Model file for the job. Use its own axes, mm. A direction names the side the tool comes from. Round coordinates to 2 decimals unless told otherwise and drop trailing zeros. Loops run counter-clockwise (first coordinate to the right, second up) from the corner with the lowest first, then second, coordinate; pieces in that order, holes last. Notation, with made-up numbers: M -30.75,16 L 14.25,16 A22 cw 14.25,53 Z; hole C 36,70 d5. An arc over 180 degrees is marked long. Use a Markdown table: item, result. Add a question column.
Q1. Pin check, flat tips, straight feed: pin 1 (6 mm diameter, centred on x = 5, z = 50, fed in from -Y); pin 2 (0.6 mm diameter, centred on x = 1, y = 51.5, fed in from -Z); pin 3 (5 mm diameter, centred on y = 97, z = 70.56, fed in from +X). Stop position of each tip, or through.
Q2. Cut at A-A (x = 6). Give the cut face in (y, z).
Q3. Cut at D-D (z = 78.5). Give the cut face in (x, y), plus the area to 3 significant figures.
Q4. Probe line 1 (Y direction, x = 1, z = 70.5); line 2 (Y direction, x = 1.5, z = 53); line 3 (Z direction, x = 6, y = 101). List the from-to ranges inside material, lowest first. Write a range as from..to.
Q5. Cut at B-B (x = 10.5). Give the cut face in (y, z).
Q6. Mould opens along Y. For faces 1 (the face through (3.2, 64.903, 53.5)), 2 (the face through (1, 109.003, 62)), 3 (the face through (5.19, 70.99, 54.22)) say: +Y half, -Y half, draft (parallel to the pull), parting line (faces both ways), or undercut.
Q7. Cut at C-C (y = 74.5). Give the cut face in (x, z).
Q8. Tool access for faces 4 (the face through (0.99, 98.39, 73.22)), 5 (the face through (3.2, 97.003, 53.5)): list every direction of +Z, -Z, +X, -X, +Y, -Y with a clear straight run to the whole face (end or side of a thin tool).
Autodesk Inventor part; units mm, degrees
ref_plane "Work Plane1" through (2, 70.903, 50.5595) normal (0, 1, 0) x (-1, 0, 0)
ref_plane "YZ Plane" through (0, 0, 0) normal (1, 0, 0) x (0, 1, 0)
ref_plane "XZ Plane" through (0, 0, 0) normal (0, 1, 0) x (-1, 0, 0)
sketch "Sketch1" plane through (0, 0, 0) normal (1, 0, 0) x (0, 1, 0)
  line L0 (109.003, 50.5595) -> (32.803, 50.5595)
  line L1 (32.803, 50.5595) -> (32.803, 88.6595)
  line L2 (32.803, 88.6595) -> (109.003, 88.6595)
  line L3 (109.003, 88.6595) -> (109.003, 50.5595)
  line L4 (76.903, 50.5595) -> (97.003, 50.5595)
  line L5 (97.003, 50.5595) -> (97.003, 57.0595)
  line L6 (97.003, 57.0595) -> (76.903, 57.0595)
  line L7 (76.903, 57.0595) -> (76.903, 50.5595)
  line L8 (44.803, 50.5595) -> (64.903, 50.5595)
  line L9 (64.903, 50.5595) -> (64.903, 57.0595)
  line L10 (64.903, 57.0595) -> (44.803, 57.0595)
  line L11 (44.803, 57.0595) -> (44.803, 50.5595)
  circle A0 centre (97.003, 70.5595) radius 3
  circle A1 centre (83.403, 80.5595) radius 3
  line L12 (70.903, 88.6595) -> (70.903, 50.5595) construction
  circle A2 centre (44.803, 70.5595) radius 3
  circle A3 centre (58.403, 80.5595) radius 3
  point P0 (0, 0)
  dimension "d0" = 76.2
  dimension "d1" = 38.1
  dimension "d2" = 6.5
  dimension "d4" = 12
  dimension "d5" = 12
  dimension "d6" = 12
  dimension "d7" = 6
  dimension "d8" = 6
  dimension "d9" = 20
  dimension "d10" = 30
  dimension "d11" = 12.5
  dimension "d12" = 26.1
extrude "Extrusion1" add sketch "Sketch1" along normal blind 2 contours L0 L5 L6 L7 L9 L10 L11 L1 L2 L3
ref_plane "Work Plane1" through (2, 70.903, 50.5595) normal (0, 1, 0) x (-1, 0, 0)
sketch "Sketch2" plane through (0, 109.003, 88.6595) normal (0, 1, 0) x (1, 0, 0)
  line L0 (0, 38.1) -> (0, 0)
  line L1 (0, 0) -> (2, 0)
  line L2 (2, 38.1) -> (2, 0)
  line L3 (0, 38.1) -> (2, 38.1)
  circle A0 centre (6, 38.1) radius 6
  line L4 (0, 38.1) -> (2, 38.1)
  line L5 (0, 38.1) -> (2, 38.1)
  circle A1 centre (6, 38.1) radius 3.75
  point P0 (0, 88.6595)
  point P1 (1.2193, 34.4744)
  point P2 (0, 38.1)
  dimension "d15" = 0
  dimension "d16" = 12
  dimension "d18" = 7.5
  dimension "d23" = 4
extrude "Extrusion2" add sketch "Sketch2" against normal up to surface (12 mm away) contours A0 L2 L3 | L3 L2 A0
mirror "Mirror1" about plane through (2, 70.903, 50.5595) normal (0, 1, 0) of "Extrusion2"
sketch "Sketch3" plane through (0, 76.903, 57.0595) normal (0, 1, 0) x (1, 0, 0)
  line L0 (0, -31.6) -> (2, -31.6)
  line L1 (0, 6.5) -> (2, 6.5)
  line L2 (0, 6.5) -> (2, 6.5)
  line L3 (0, 6.5) -> (0, -31.6)
  line L4 (2, 2.0279) -> (2, -31.6)
  arc A0 (2, 2.0279) -> (0, 6.5) centre (6, 6.5) ccw
  circle A1 centre (6, 6.5) radius 3.75
  circle A2 centre (6, 6.5) radius 3.75
  line L5 (0, 6.5) -> (0, -31.6)
  line L6 (0, -31.6) -> (2, -31.6)
  line L7 (2, 2.0279) -> (2, -31.6)
  arc A3 (2, 2.0279) -> (0, 6.5) centre (6, 6.5) ccw
  line L8 (2, 6.5) -> (2, 0)
  point P0 (0, 57.0595)
extrude "Extrusion3" add sketch "Sketch3" against normal up to surface (12 mm away) contours A0 L8 L1
equation "\"d5\" = d4"
equation "\"d6\" = d4"
equation "\"d8\" = d7"
properties part number "zawias-lewy" material "Stainless Steel"
Checked values:
| question | item | result |
|---|---|---|
| 1 | pin 1 | stops at y = 32.8 |
| 1 | pin 2 | stops at z = 57.06 |
| 1 | pin 3 | passes through |
| 2 | outline | M 32.8,44.56 L 44.8,44.56 L 44.8,46.81 L 32.8,46.81 Z; M 32.8,54.31 L 44.8,54.31 L 44.8,56.56 L 32.8,56.56 Z; M 64.9,44.56 L 76.9,44.56 L 76.9,46.81 L 64.9,46.81 Z; M 64.9,54.31 L 76.9,54.31 L 76.9,56.56 L 64.9,56.56 Z; M 97,44.56 L 109,44.56 L 109,46.81 L 97,46.81 Z; M 97,54.31 L 109,54.31 L 109,56.56 L 97,56.56 Z |
| 3 | outline | M 0,32.8 L 2,32.8 L 2,56.22 L 0,56.22 Z; M 0,60.58 L 2,60.58 L 2,81.22 L 0,81.22 Z; M 0,85.58 L 2,85.58 L 2,109 L 0,109 Z |
| 3 | area | 135 mm^2 |
| 4 | line 1 | y = 32.8..41.8, 47.8..94, 100..109 |
| 4 | line 2 | y = 32.8..44.8, 64.9..76.9, 97..109 |
| 4 | line 3 | z = 44.56..46.81, 54.31..56.56 |
| 5 | outline | M 32.8,46.59 L 44.8,46.59 L 44.8,54.53 L 32.8,54.53 Z; M 64.9,46.59 L 76.9,46.59 L 76.9,54.53 L 64.9,54.53 Z; M 97,46.59 L 109,46.59 L 109,54.53 L 97,54.53 Z |
| 6 | face 1 | undercut |
| 6 | face 2 | +Y half |
| 6 | face 3 | draft |
| 7 | outline | M 0,50.56 A6 ccw long 2,55.03 L 2,88.66 L 0,88.66 Z; hole C 6,50.56 d7.5 |
| 8 | face 4 | +X, -X |
| 8 | face 5 | -Z, +X, -X |
